Autodesk Fusion 360 part; units mm, degrees
sketch "Sketch1" plane through (0, 0, 0) normal (0, 1, 0) x (1, 0, 0)
  line L0 (0, 0) -> (22, 0)
  line L1 (22, 0) -> (22, -19)
  line L2 (22, -19) -> (0, -19)
  line L3 (0, -19) -> (0, 0)
  line L4 (0, -9.5) -> (22, -9.5) construction
  line L5 (17.5, -13.2528) -> (17.5, -5.7472)
  line L6 (17.5, -5.7472) -> (11, -1.9944)
  line L7 (11, -1.9944) -> (4.5, -5.7472)
  line L8 (4.5, -5.7472) -> (4.5, -13.2528)
  line L9 (4.5, -13.2528) -> (11, -17.0056)
  line L10 (11, -17.0056) -> (17.5, -13.2528)
  line L11 (17.5, -13.2528) -> (17.5, -19)
  line L12 (4.5, -13.2528) -> (4.5, -19)
  circle A0 centre (11, -9.5) radius 4.2
  point P0 (11, -9.5)
  dimension "d1" = 19
  dimension "d2" = 22
  dimension "d3" = 13
  dimension "d4" = 8.4
extrude "Extrude1" add sketch "Sketch1" along normal blind 30
extrude "Extrude2" cut sketch "Sketch1" along normal blind 7 from surface at 11 contours L2 L9 L10 L11 L12 | L5 L6 L7 L8 L9 L10
chamfer "Chamfer1" distance 0.4 angle 45 18 edges at (0, 15, 19) (0, 15, 0) (22, 15, 19) (22, 15, 0) (22, 30, 9.5) (11, 30, 19) (0, 30, 9.5) (11, 30, 0) (22, 0, 9.5) (11, 0, 19) (11, 0, 0) (0, 0, 9.5) (4.5, 14.5, 19) (17.5, 14.5, 19) (7.0842, 0, 7.9812) (7.0842, 30, 7.9812) (11, 18, 19) (11, 11, 19)
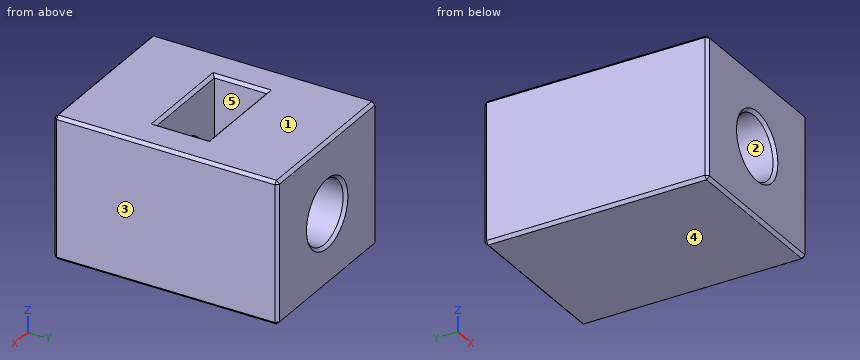
Here's how the part is built. I have some questions about the finished solid (model axes, mm). Face numbers are marked on the shaded views. A direction names the side the tool comes from. Round coordinates to 2 decimals unless told otherwise and drop trailing zeros. Loops run counter-clockwise (first coordinate to the right, second up) from the corner with the lowest first, then second, coordinate; pieces in that order, holes last.
1. If we section it at A-A on y = 24.25: Write out the boundary of the cut face in (x, z), plus the area to 3 significant figures.
Answer list:
outline: (0, 0.4) - (0.4, 0) - (21.6, 0) - (22, 0.4) - (22, 18.6) - (21.6, 19) - (0.4, 19) - (0, 18.6) - close; hole circle Ø8.4 at (11, 9.5)
area: 362 mm2
2. If we section it at B-B on z = 9.5: Write out the boundary of the cut face in (x, y).
Answer list:
outline: (0, 0.4) - (0.4, 0) - (6.4, 0) - (6.8, 0.4) - (6.8, 11) - (4.5, 11) - (4.5, 18) - (6.8, 18) - (6.8, 29.6) - (6.4, 30) - (0.4, 30) - (0, 29.6) - close; (15.2, 0.4) - (15.6, 0) - (21.6, 0) - (22, 0.4) - (22, 29.6) - (21.6, 30) - (15.6, 30) - (15.2, 29.6) - (15.2, 18) - (17.5, 18) - (17.5, 11) - (15.2, 11) - close
3. Which directions (+Z, -Z, +X, -X, +Y, -Y) give clear straight access to the entire face, cutting with the end or side of a thin tool? Please do the marked faces 4 and 5.
Answer list:
face 4: -Z, +X, -X, +Y, -Y
face 5: +Z
4. If I drill on line 1 along Z through (x, y) = (11, 25.25); line 2 along X through (y, z) = (14.75, 16.25); line 3 along X through (y, z) = (24.25, 9.5), over which ranges is the centre line in solid material (lowest first)?
Answer list:
line 1: z = 0 to 5.3, 13.7 to 19
line 2: x = 0 to 4.5, 17.5 to 22
line 3: x = 0 to 6.8, 15.2 to 22
5. We'd pull the mould along Z, two halves only. Please class the marked faces 1, 2 and 3: +Z half, -Z half, draft (parallel to the pull), parting line (faces both ways), or undercut.
Answer list:
face 1: +Z half
face 2: undercut
face 3: draft
6. For P1, Ø10.5, axis at x = 13.5, z = 14, coming from the -Y side, with a flat end and sliding along its axis, tell me the tip position at first contact or that it passes through.
Answer list:
P1: stops at y = 0
7. If we section it at D-D on x = 11.75: Count the separate pieces of the cut face and the enclosed holes in it, plus the area to 3 significant figures.
Answer list:
separate pieces: 3
enclosed holes: 0
area: 263 mm2
8. If we section it at C-C on z = 2.5: Write out the boundary of the cut face in (x, y).
Answer list:
outline: (0, 0.4) - (0.4, 0) - (21.6, 0) - (22, 0.4) - (22, 29.6) - (21.6, 30) - (0.4, 30) - (0, 29.6) - close; hole (10.12, 11) - (11.88, 11) - (11.88, 18) - (10.12, 18) - close
